Geometry check sheet. Reference: the model listing, model coordinates, mm. A direction names the side the tool comes from. Give positions to 0.01 mm unless a question says otherwise; leave off trailing zeros. Write each loop counter-clockwise with the first axis right and the second up, starting at its lowest first coordinate (ties: lowest second). Pieces come first, ordered by that corner, then holes. Notation, with made-up numbers: (27.5, 58.25) - (36.5, 58.25) arc R16 cw to (36.5, 87.25) - close; hole circle Ø11 at (36.25, 11.25). An arc over 180 degrees is marked (long way). Use a Markdown table: item, result.
```python
from build123d import *

# Parameters (mm, degrees)
F1_DEPTH = 150
F2_W     = 50
F2_H     = 12
F3_DEPTH = 60
F4_W     = 126
F4_H     = 15.081386
F5_DEPTH = 48


with BuildPart() as f1:
    # F0 (on Right) → F1 (new body)
    with BuildSketch(Plane.YZ):
        Polygon((0, 32), (0, 0), (60, 0), (60, 48), (30, 48), (30, 32), align=None)
    extrude(amount=F1_DEPTH)

    # F2 (on Front) → F3 (cut)
    with BuildSketch(Plane.XZ):
        with Locations((75, 6)):
            Rectangle(F2_W, F2_H)
    extrude(amount=-F3_DEPTH, mode=Mode.SUBTRACT)

    # F4 (on Top) → F5 (cut)
    with BuildSketch(Plane.XY):
        with Locations((75, 52.540693)):
            Rectangle(F4_W, F4_H)
    extrude(amount=F5_DEPTH, mode=Mode.SUBTRACT)


solid = f1.part
```
1) Section check A-A on z = 6. Record the boundary of the cut face in (x, y).
Working result:
| item | result |
|---|---|
| outline | (0, 0) - (50, 0) - (50, 45) - (12, 45) - (12, 60) - (0, 60) - close; (100, 0) - (150, 0) - (150, 60) - (138, 60) - (138, 45) - (100, 45) - close |
2) Section check B-B on y = 52.5. Record the boundary of the cut face in (x, z), then the cut area to 3 significant figures.
Working result:
| item | result |
|---|---|
| outline | (0, 0) - (12, 0) - (12, 48) - (0, 48) - close; (138, 0) - (150, 0) - (150, 48) - (138, 48) - close |
| area | 1,150 mm² |
3) Depth check by flat-ended pin: P1, Ø14.5, axis at x = 103, z = 36, coming from the +Y side; P2, Ø16.5, axis at y = 53.5, z = 22, coming from the -X side; P3, Ø22.5, axis at x = 85.5, y = 26, coming from the -Z side. Enter the tip coordinate at first touch or a pass-through.
Working result:
| item | result |
|---|---|
| P1 | stops at y = 45 |
| P2 | stops at x = 0 |
| P3 | stops at z = 12 |
4) Material ranges on L1, parallel to X at y = 47, z = 21; L2, parallel to X at y = 35, z = 10; L3, parallel to Z at x = 111.5, y = 3.5, recorded low to high. Write a range as from..to.
Working result:
| item | result |
|---|---|
| L1 | x = 0..12, 138..150 |
| L2 | x = 0..50, 100..150 |
| L3 | z = 0..32 |
5) Set-up check for faces 1 (the flat face through (74, 30, 40)), 2 (the flat face through (74, 39, 48)), 3 (the flat face through (12, 52, 24)), 4 (the flat face through (75, 22, 12)): record each of +Z, -Z, +X, -X, +Y, -Y from which the full face is reachable in a straight line by a thin tool's end or side.
Working result:
| item | result |
|---|---|
| face 1 | +Z, +X, -X, -Y |
| face 2 | +Z, +X, -X, +Y, -Y |
| face 3 | +Z, -Z, +Y |
| face 4 | -Z, +Y, -Y |
6) Section check C-C on y = 24. Record the boundary of the cut face in (x, z).
Working result:
| item | result |
|---|---|
| outline | (0, 0) - (50, 0) - (50, 12) - (100, 12) - (100, 0) - (150, 0) - (150, 32) - (0, 32) - close |
7) Section check D-D on x = 16.5. Record the boundary of the cut face in (y, z).
Working result:
| item | result |
|---|---|
| outline | (0, 0) - (45, 0) - (45, 48) - (30, 48) - (30, 32) - (0, 32) - close |
8) Mould release check, pull along X, two halves, no side actions. Record for faces 5 (the flat face through (0, 30, 19)), 6 (the flat face through (100, 22, 6)), 7 (the flat face through (74, 0, 16)): pulls with the +X half, pulls with the -X half, needs draft (parallel to the pull), parting line crosses it, or undercut.
Working result:
| item | result |
|---|---|
| face 5 | pulls with the -X half |
| face 6 | undercut |
| face 7 | needs draft |
